Read the model definition and answer for the solid it produces. Units are mm, in the model's axes. Give positions to 0.01 mm unless a question says otherwise; leave off trailing zeros. Return JSON: item names as keys, results as strings. Group by question number.
```python
from build123d import *

# Parameters (mm, degrees)
BOSS_EXTRUDE1_DEPTH     = 5
CUT_EXTRUDE1_DEPTH      = 0.1
CUT_EXTRUDE2_DEPTH      = 194.597682063
CUT_EXTRUDE2_DEPTH_BACK = 194.597682063
SKETCH3_W               = 6
SKETCH3_H               = 162
SKETCH3_W_2             = 116.5
SKETCH3_H_2             = 5
CUT_EXTRUDE4_DEPTH      = 186.790372463
CUT_EXTRUDE4_DEPTH_BACK = 186.790372463
SKETCH7_R               = 1.5


with BuildPart() as part:
    # Sketch1 → Boss-Extrude1 (new body)
    with BuildSketch(Plane(origin=(0, 0, 0), x_dir=(1, 0, 0), z_dir=(0, 1, 0))):
        Polygon((-58.25, 125), (58.25, 125), (58.25, 81), (147.75, 81), (147.75, -81), (58.25, -81), (58.25, -125), (-58.25, -125), (-58.25, -81), (-147.75, -81), (-147.75, 81), (-58.25, 81), align=None)
    extrude(amount=BOSS_EXTRUDE1_DEPTH)

    # Sketch2 → Cut-Extrude1 (cut)
    with BuildSketch(Plane.XZ):
        Polygon((-103, 65), (-82.5, 65), (-82.5, 70), (-123.5, 70), (-123.5, 65), align=None)
        Polygon((123.5, 70), (123.5, 65), (103, 65), (82.5, 65), (82.5, 70), align=None)
        Polygon((-123.5, -70), (-123.5, -65), (-103, -65), (-82.5, -65), (-82.5, -70), align=None)
        Polygon((82.5, -70), (123.5, -70), (123.5, -65), (103, -65), (82.5, -65), align=None)
    extrude(amount=-CUT_EXTRUDE1_DEPTH, mode=Mode.SUBTRACT)

    # Sketch3 → Cut-Extrude2 (cut, two sides: drawn at the far end of the back side and taken through both)
    with BuildSketch(Plane(origin=(0, 5, 0), x_dir=(1, 0, 0), z_dir=(0, 1, 0)).offset(-CUT_EXTRUDE2_DEPTH_BACK)):
        with Locations((-144.75, 0)):
            Rectangle(SKETCH3_W, SKETCH3_H)
        with Locations((144.75, 0)):
            Rectangle(SKETCH3_W, SKETCH3_H)
        with Locations((0, 122.5)):
            Rectangle(SKETCH3_W_2, SKETCH3_H_2)
        with Locations((0, -122.5)):
            Rectangle(SKETCH3_W_2, SKETCH3_H_2)
    extrude(amount=CUT_EXTRUDE2_DEPTH + CUT_EXTRUDE2_DEPTH_BACK, mode=Mode.SUBTRACT)

    # Sketch7 → Cut-Extrude4 (cut, two sides: drawn at the far end of the back side and taken through both)
    with BuildSketch(Plane(origin=(0, 5, 0), x_dir=(1, 0, 0), z_dir=(0, 1, 0)).offset(-CUT_EXTRUDE4_DEPTH_BACK)):
        with Locations(Location((25, -65, 0), (0, 0, 270))):
            Circle(SKETCH7_R)
        with Locations(Location((35, -65, 0), (0, 0, 90))):
            Circle(SKETCH7_R)
        with Locations(Location((-35, -65, 0), (0, 0, 270))):
            Circle(SKETCH7_R)
        with Locations(Location((-25, -65, 0), (0, 0, 90))):
            Circle(SKETCH7_R)
        with Locations(Location((-25, 65, 0), (0, 0, 270))):
            Circle(SKETCH7_R)
        with Locations(Location((-35, 65, 0), (0, 0, 90))):
            Circle(SKETCH7_R)
        with Locations(Location((35, 65, 0), (0, 0, 270))):
            Circle(SKETCH7_R)
        with Locations(Location((25, 65, 0), (0, 0, 90))):
            Circle(SKETCH7_R)
    extrude(amount=CUT_EXTRUDE4_DEPTH + CUT_EXTRUDE4_DEPTH_BACK, mode=Mode.SUBTRACT)


solid = part.part
```
1. Flat-ended cylindrical pins translate along their axes: P1, Ø1, axis at x = 97, y = 1.5, coming from the +Z side; P2, Ø2.5, axis at x = -120.5, y = 1.5, coming from the -Z side; P3, Ø2.5, axis at x = -35, z = 65, coming from the +Y side. Find the tip coordinate at first contact, or state that the pin passes through.
2. Find section A-A (y = 3.75). State how many separate pieces and enclosed holes the cut face has, and give its area (3 significant figures).
3. Straight lines are drawn through the part: line 1 along X through (y, z) = (0.8, -66); line 2 along Z through (x, y) = (108, 1.5); line 3 along Z through (x, y) = (24, 1.3). For each, find the intervals that lie inside material, in ascending order.
Result:
{
 "1": {"P1": "stops at z = 81", "P2": "stops at z = -81", "P3": "passes through"},
 "2": {"separate pieces": "1", "enclosed holes": "8", "area": "55,000 mm2"},
 "3": {"line 1": "x = -141.75 to -36.12, -33.88 to -26.12, -23.88 to 23.88, 26.12 to 33.88, 36.12 to 141.75", "line 2": "z = -81 to 81", "line 3": "z = -120 to -66.12, -63.88 to 63.88, 66.12 to 120"}
}
